from build123d import *

# Parameters (mm, degrees)
SKETCH_R        = 6.5
SKETCH_R_2      = 2
PAD_DEPTH       = 5
SKETCH001_R     = 5.5
SKETCH001_R_2   = 2.85
POCKET_DEPTH    = 0.5
SKETCH002_R     = 5.5
SKETCH002_R_2   = 2.85
POCKET001_DEPTH = 0.5


with BuildPart() as part:
    # Sketch → Pad (new body)
    with BuildSketch(Plane.XY):
        Circle(SKETCH_R)
        Circle(SKETCH_R_2, mode=Mode.SUBTRACT)
    extrude(amount=PAD_DEPTH)

    # Sketch001 (on Face4 of Pad) → Pocket (cut)
    with BuildSketch(Plane.XY.offset(5)):
        Circle(SKETCH001_R)
        Circle(SKETCH001_R_2, mode=Mode.SUBTRACT)
    extrude(amount=-POCKET_DEPTH, mode=Mode.SUBTRACT)

    # Sketch002 (on Face2 of Pocket) → Pocket001 (cut)
    with BuildSketch(Plane(origin=(0, 0, 0), x_dir=(1, 0, 0), z_dir=(0, 0, -1))):
        Circle(SKETCH002_R)
        Circle(SKETCH002_R_2, mode=Mode.SUBTRACT)
    extrude(amount=-POCKET001_DEPTH, mode=Mode.SUBTRACT)


solid = part.part
Input: part model. Units: mm. Frame: model coordinates. A direction names the side the tool comes from. Give positions to 0.01 mm unless a question says otherwise; leave off trailing zeros. Order: outer loops, then holes, each group sorted by start corner. A loop starts at its lowest first (then second) coordinate and runs counter-clockwise, first axis right, second up.
Q1. Set-up query: faces 4 (the flat face through (2.4, -2.4, 4.5)), 5 (the cylindrical face through (-1.19, 5.37, 0.25)), 6 (the flat face through (-5, 3, 0)). Return all of +Z, -Z, +X, -X, +Y, -Y with unobstructed straight access to the full face (end or side cutting, diameter ignored); none if empty.
Checked values:
face 4: +Z
face 5: -Z
face 6: -Z, +X, -X, +Y, -Y
Q2. Section D-D on x = 4.25. Output: boundary loops of the cut face in (y, z), and give its area (3 significant figures).
Checked values:
outline: (-4.92, 0) - (-3.49, 0) - (-3.49, 0.5) - (3.49, 0.5) - (3.49, 0) - (4.92, 0) - (4.92, 5) - (3.49, 5) - (3.49, 4.5) - (-3.49, 4.5) - (-3.49, 5) - (-4.92, 5) - close
area: 42.2 mm2
Q3. Ray query, probe 1 along Y at (x, z) = (0, 4.8); probe 2 along Y at (x, z) = (0, 2.5); probe 3 along Y at (x, z) = (-2.5, 0.35). Return the intervals inside material, ascending.
Checked values:
probe 1: y = -6.5 to -5.5, -2.85 to -2, 2 to 2.85, 5.5 to 6.5
probe 2: y = -6.5 to -2, 2 to 6.5
probe 3: y = -6 to -4.9, -1.37 to 1.37, 4.9 to 6
Q4. Section C-C on y = -5.25. Output: boundary loops of the cut face in (x, z), and give its area (3 significant figures).
Checked values:
outline: (-3.83, 0) - (-1.64, 0) - (-1.64, 0.5) - (1.64, 0.5) - (1.64, 0) - (3.83, 0) - (3.83, 5) - (1.64, 5) - (1.64, 4.5) - (-1.64, 4.5) - (-1.64, 5) - (-3.83, 5) - close
area: 35.0 mm2
Q5. Draft query along Y for faces 1 (the cylindrical face through (-5.158, -3.955, 2.465)), 2 (the cylindrical face through (-2.262, 1.734, 0.246)), 3 (the flat face through (-5, 3, 5)). Return one class per face: +Y half, -Y half, draft (parallel to the pull), parting line (faces both ways), or undercut.
Checked values:
face 1: parting line
face 2: undercut
face 3: draft
Q6. Contact query for flat-ended pins moving along their axis: pin 1 Ø1 at (x, y) = (0, -0.5) entering from +Z; pin 2 Ø1.5 at (x, z) = (-2.5, 2.5) entering from +Y; pin 3 Ø1.5 at (x, y) = (2.5, -3.5) entering from +Z. Output: stop coordinate, or through.
Checked values:
pin 1: passes through
pin 2: stops at y = 6.26
pin 3: stops at z = 4.5
Q7. Section A-A on y = 0. Output: boundary loops of the cut face in (x, z).
Checked values:
outline: (-6.5, 0) - (-5.5, 0) - (-5.5, 0.5) - (-2.85, 0.5) - (-2.85, 0) - (-2, 0) - (-2, 5) - (-2.85, 5) - (-2.85, 4.5) - (-5.5, 4.5) - (-5.5, 5) - (-6.5, 5) - close; (2, 0) - (2.85, 0) - (2.85, 0.5) - (5.5, 0.5) - (5.5, 0) - (6.5, 0) - (6.5, 5) - (5.5, 5) - (5.5, 4.5) - (2.85, 4.5) - (2.85, 5) - (2, 5) - close
